Can you work these out from the model? Positions are in its coordinate system, mm. Face numbers are marked on the shaded views. A direction names the side the tool comes from. Give positions to 0.01 mm unless a question says otherwise; leave off trailing zeros. Order: outer loops, then holes, each group sorted by start corner. A loop starts at its lowest first (then second) coordinate and runs counter-clockwise, first axis right, second up. Notation, with made-up numbers: (73, 20) - (105, 20) arc R22 cw to (105, 38) - close; hole circle Ø8 at (-1.5, 79). An arc over 180 degrees is marked (long way). Return JSON: item names as keys, results as strings.
```python
from build123d import *

# Parameters (mm, degrees)
F0_W     = 107.0926934481
F0_H     = 38.6895574629
F0_W_2   = 38.9990732074
F1_DEPTH = 40.386
F2_R     = 22.3315998305
F2_R_2   = 21.9640238971
F3_DEPTH = 61.214
F4_W     = 69.3601816893
F4_H     = 29.5533258468
F4_W_2   = 51.8825063482
F4_H_2   = 14.1199231148
F5_DEPTH = 100.076
F7_DEPTH = 65.786


with BuildPart() as f1:
    # F0 (on Front) → F1 (new body)
    with BuildSketch(Plane.XZ):
        with BuildLine():
            ThreePointArc((-5.3047918225, 21.9756681472), (-1.760973589, 31.599753627), (-0.5576112402, 41.784722358))
            ThreePointArc((-0.5576112402, 41.784722358), (-62.1276824989, 81.6689250655), (-73.3553990722, 9.1736722487))
            Line((-73.3553990722, 9.1736722487), (-73.3553990722, 21.9756681472))
            Line((-73.3553990722, 21.9756681472), (-5.3047918225, 21.9756681472))
        make_face()
        with BuildLine():
            Line((-73.3553990722, 21.9756681472), (-73.3553990722, 9.1736722487))
            ThreePointArc((-73.3553990722, 9.1736722487), (-36.1809302997, -1.1651102493), (-5.3047918225, 21.9756681472))
            Line((-5.3047918225, 21.9756681472), (-73.3553990722, 21.9756681472))
        make_face()
        with BuildLine():
            ThreePointArc((-5.3047918225, 21.9756681472), (-36.1809302997, -1.1651102493), (-73.3553990722, 9.1736722487))
            Line((-73.3553990722, 9.1736722487), (-73.3553990722, -65.3079673648))
            Line((-73.3553990722, -65.3079673648), (39.6181046963, -65.3079673648))
            Line((39.6181046963, -65.3079673648), (39.6181046963, -48.594083637))
            Line((39.6181046963, -48.594083637), (-67.4745887518, -48.594083637))
            Line((-67.4745887518, -48.594083637), (-67.4745887518, -9.9045261741))
            Line((-67.4745887518, -9.9045261741), (39.6181046963, -9.9045261741))
            Line((39.6181046963, -9.9045261741), (39.6181046963, 21.9756681472))
            Line((39.6181046963, 21.9756681472), (-5.3047918225, 21.9756681472))
        make_face()
        with Locations((-13.9282420278, -29.2493049055)):
            Rectangle(F0_W, F0_H)
        with Locations((59.1176413, -29.2493049055)):
            Rectangle(F0_W_2, F0_H)
    extrude(amount=F1_DEPTH)

    # F2 (on Front) → F3 (join)
    with BuildSketch(Plane.XZ):
        with Locations((-47.0310002565, 48.6432611942)):
            Circle(F2_R)
        with Locations((-47.0310002565, 48.6432611942)):
            Circle(F2_R_2, mode=Mode.SUBTRACT)
    extrude(amount=F3_DEPTH)

    # F4 (on Front) → F5 (join)
    with BuildSketch(Plane.XZ):
        with Locations((-34.6800908446, -40.3450904414)):
            Rectangle(F4_W, F4_H)
        with Locations((-34.5529275946, -40.5092760921)):
            Rectangle(F4_W_2, F4_H_2, mode=Mode.SUBTRACT)
    extrude(amount=F5_DEPTH)

    # F6 (on Front) → F7 (join)
    with BuildSketch(Plane.XZ):
        with BuildLine():
            ThreePointArc((71.5539108322, -62.4836369352), (89.0145397665, -51.3617017106), (95.8118023382, -31.8074636161))
            ThreePointArc((95.8118023382, -31.8074636161), (89.0145397665, -12.2532255217), (71.5539108322, -1.1312902971))
            ThreePointArc((71.5539108322, -1.1312902971), (39.8321670237, -31.8074636161), (71.5539108322, -62.4836369352))
        make_face()
        with BuildLine():
            ThreePointArc((71.5539108322, -1.1312902971), (89.0145397665, -12.2532255217), (95.8118023382, -31.8074636161))
            ThreePointArc((95.8118023382, -31.8074636161), (89.0145397665, -51.3617017106), (71.5539108322, -62.4836369352))
            ThreePointArc((71.5539108322, -62.4836369352), (92.5896637981, -53.1443080624), (101.2189763841, -31.8074636161))
            ThreePointArc((101.2189763841, -31.8074636161), (92.5896637981, -10.4706191698), (71.5539108322, -1.1312902971))
        make_face()
        with BuildLine():
            ThreePointArc((71.5539108322, -62.4836369352), (39.8321670237, -31.8074636161), (71.5539108322, -1.1312902971))
            ThreePointArc((71.5539108322, -1.1312902971), (32.7612725987, -31.8074636161), (71.5539108322, -62.4836369352))
        make_face()
    extrude(amount=-F7_DEPTH)


solid = f1.part
```
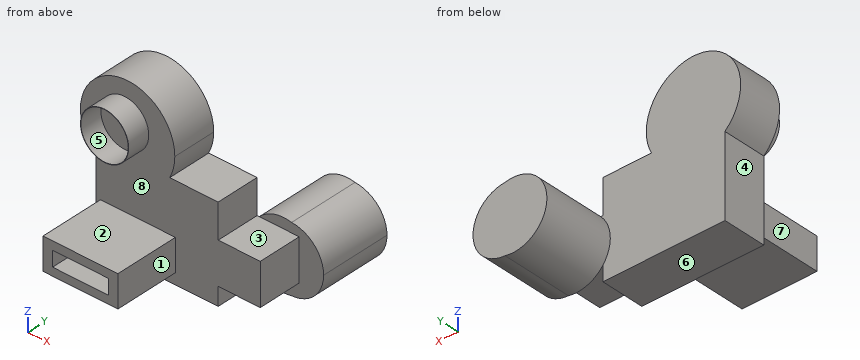
1. Suppose I cut it at C-C (x = -38). List the corners of the cut face in (y, z) for me, plus the area to 3 significant figures.
Checks:
{"outline": "(-100.08, -55.12) - (-40.39, -55.12) - (-40.39, -65.31) - (0, -65.31) - (0, 85.04) - (-40.39, 85.04) - (-40.39, 69.07) - (-61.21, 69.07) - (-61.21, 68.66) - (-40.39, 68.66) - (-40.39, 28.62) - (-61.21, 28.62) - (-61.21, 28.22) - (-40.39, 28.22) - (-40.39, -25.57) - (-100.08, -25.57) - (-100.08, -33.45) - (-40.39, -33.45) - (-40.39, -47.57) - (-100.08, -47.57) - close", "area": "7,010 mm^2"}
2. For pin 1 Ø4 at (x, y) = (13, -17) entering from +Z; pin 2 Ø15.5 at (x, y) = (-25.5, -80) entering from -Z; pin 3 Ø5 at (x, z) = (-47, -10.5) entering from +Y, each with a flat end and sliding along its axis, tell me the tip position at first contact or that it passes through.
Checks:
{"pin 1": "z = 21.98", "pin 2": "z = -55.12", "pin 3": "y = 0"}
3. If I drill on L1, parallel to Z at x = -43, y = -54; L2, parallel to Y at x = -39.5, z = 78; L3, parallel to X at y = -35, z = -29.5, over which ranges is the centre line in solid material (lowest first)? Write a range as [from, to].
Checks:
{"L1": "[-55.12, -47.57], [-33.45, -25.57], [26.68, 27.05], [70.23, 70.61]", "L2": "[-40.39, 0]", "L3": "[-73.36, 78.62]"}
4. Thinking about a two-plate mould opening in Z: for the marked faces 6, 7 and 8, which applies, +Z half, -Z half, draft (parallel to the pull), parting line (faces both ways), or undercut?
Checks:
{"face 6": "-Z half", "face 7": "draft", "face 8": "undercut"}
5. On a 3-axis mill with a long thin cutter (end or side, diameter ignored), from which of +Z, -Z, +X, -X, +Y, -Y can I reach the whole of each face in a straight line? I mean the marked faces 1, 2, 3, 4 and 5. Say none if no direction works.
Checks:
{"face 1": "+Z, -Z, +X, -Y", "face 2": "+X, -X, -Y", "face 3": "+Z, +X, -Y", "face 4": "-Z, -X, +Y, -Y", "face 5": "-Y"}
6. Suppose I cut it at B-B (y = -14.5). List the corners of the cut face in (x, z) for me, plus the area to 3 significant figures.
Checks:
{"outline": "(-73.36, -65.31) - (39.62, -65.31) - (39.62, -48.59) - (78.62, -48.59) - (78.62, -9.9) - (39.62, -9.9) - (39.62, 21.98) - (-5.3, 21.98) arc R43.7 ccw (long way) to (-73.36, 9.17) - close", "area": "16,100 mm^2"}
7. Suppose I cut it at D-D (x = 57). List the corners of the cut face in (y, z) for me, plus the area to 3 significant figures.
Checks:
{"outline": "(-40.39, -48.59) - (0, -48.59) - (0, -62.48) - (65.79, -62.48) - (65.79, -1.14) - (0, -1.14) - (0, -9.9) - (-40.39, -9.9) - close", "area": "5,600 mm^2"}
8. Suppose I cut it at A-A (z = -5.5). List the corners of the cut face in (x, y) for me, plus the area to 3 significant figures.
Checks:
{"outline": "(-73.36, -40.39) - (39.62, -40.39) - (39.62, 0) - (-73.36, 0) - close; (46.92, 0) - (86.34, 0) - (86.34, 65.79) - (46.92, 65.79) - close", "area": "7,160 mm^2"}
